from build123d import *

# Parameters (mm, degrees)
F0_W     = 250
F0_H     = 399.7749028206
F1_DEPTH = 90
F3_W     = 250
F3_H     = 413
F4_DEPTH = 4


with BuildPart() as f1:
    # F0 (on Top) → F1 (new body)
    with BuildSketch(Plane.XY):
        Polygon((-288, 0), (0, 0), (19, 0), (19, 15.7749028206), (19, 19), (0, 19), (0, 418.7749028206), (0, 437.7749028206), (-288, 437.7749028206), (-288, 19), (-307, 19), (-307, 0), align=None)
        with Locations((-144, 218.8874514103)):
            Rectangle(F0_W, F0_H, mode=Mode.SUBTRACT)
    extrude(amount=-F1_DEPTH)

    # F3 (on offset) → F4 (join)
    with BuildSketch(Plane.XY.offset(-85)):
        with Locations((-144, 225.5)):
            Rectangle(F3_W, F3_H)
    extrude(amount=F4_DEPTH)


solid = f1.part
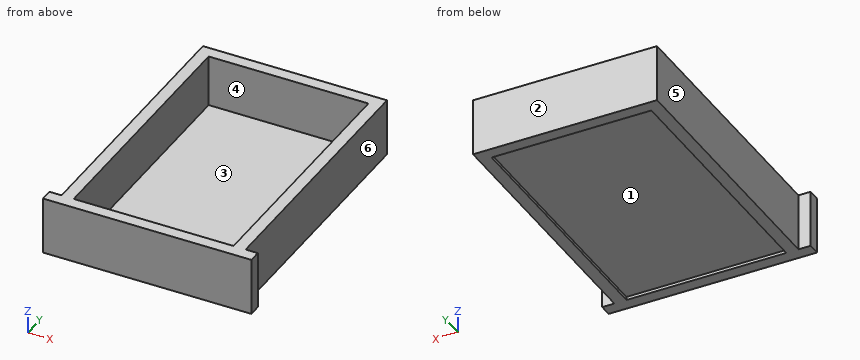
Here's how the part is built. I have some questions about the finished solid (model axes, mm). Face numbers are marked on the shaded views. A direction names the side the tool comes from. Coordinates: 2 decimals unless noted, no trailing zeros. Write each loop counter-clockwise with the first axis right and the second up, starting at its lowest first coordinate (ties: lowest second). Pieces come first, ordered by that corner, then holes.
Item 1: I want a section at A-A on x = -96. Write out the boundary of the cut face in (y, z), and give its area (3 significant figures).
Item 2: If I drill on line 1 (X direction, y = 22.5, z = -38); line 2 (Y direction, x = -233, z = -20.5); line 3 (Z direction, x = -202.5, y = 285), over which ranges is the centre line in solid material (lowest first)?
Item 3: On a 3-axis mill with a long thin cutter (end or side, diameter ignored), from which of +Z, -Z, +X, -X, +Y, -Y can I reach the whole of each face in a straight line? I mean the marked faces 1, 2 and 3. Say none if no direction works.
Item 4: Will these pins go through, and if not, where does the flat tip stop? pin 1 (1.5 mm diameter, centred on y = 296, z = -56.5, fed in from +X); pin 2 (12 mm diameter, centred on x = -65.5, y = 149, fed in from +Z); pin 3 (9.5 mm diameter, centred on x = -299.5, z = -50, fed in from +Y).
Item 5: If we mould it in two halves opening along X, with no side actions, what happens to the marked faces 4, 5 and 6? For each: +X half, -X half, draft (parallel to the pull), parting line (faces both ways), or undercut.
Item 6: I want a section at C-C on y = 130. Write out the boundary of the cut face in (x, z), and give its area (3 significant figures).
Item 7: I want a section at B-B on z = -33.5. Write out the boundary of the cut face in (x, y).
Findings below:
1. outline: (0, -90) - (19, -90) - (19, -85) - (418.77, -85) - (418.77, -90) - (437.77, -90) - (437.77, 0) - (418.77, 0) - (418.77, -81) - (19, -81) - (19, 0) - (0, 0) - close
1. area: 5,020 mm2
2. line 1: x = -288 to -269, -19 to 0
2. line 2: y = 0 to 19, 418.77 to 437.77
2. line 3: z = -85 to -81
3. face 1: -Z
3. face 2: +Z, -Z, +X, -X, +Y
3. face 3: +Z
4. pin 1: stops at x = 0
4. pin 2: stops at z = -81
4. pin 3: stops at y = 19
5. face 4: undercut
5. face 5: -X half
5. face 6: +X half
6. outline: (-288, -90) - (-269, -90) - (-269, -85) - (-19, -85) - (-19, -90) - (0, -90) - (0, 0) - (-19, 0) - (-19, -81) - (-269, -81) - (-269, 0) - (-288, 0) - close
6. area: 4,420 mm2
7. outline: (-307, 0) - (19, 0) - (19, 19) - (0, 19) - (0, 437.77) - (-288, 437.77) - (-288, 19) - (-307, 19) - close; hole (-269, 19) - (-19, 19) - (-19, 418.77) - (-269, 418.77) - close
